```python
from build123d import *

# Parameters (mm, degrees)
ESQUISSE1_W             = 54
ESQUISSE1_H             = 14
ESQUISSE1_W_2           = 50.4
ESQUISSE1_H_2           = 10.4
BOSS_EXTRU_1_DEPTH      = 10
ESQUISSE2_W             = 54
ESQUISSE2_H             = 14
BOSS_EXTRU_2_DEPTH      = 1
ENL_V_MAT_EXTRU_1_DEPTH = 1
ESQUISSE4_W             = 50.4
ESQUISSE4_H             = 10
ENL_V_MAT_EXTRU_2_DEPTH = 1.8


with BuildPart() as part:
    # Esquisse1 → Boss.-Extru.1 (new body)
    with BuildSketch(Plane(origin=(0, 0, 0), x_dir=(1, 0, 0), z_dir=(0, 1, 0))):
        Rectangle(ESQUISSE1_W, ESQUISSE1_H)
        Rectangle(ESQUISSE1_W_2, ESQUISSE1_H_2, mode=Mode.SUBTRACT)
    extrude(amount=BOSS_EXTRU_1_DEPTH)

    # Esquisse2 → Boss.-Extru.2 (add)
    with BuildSketch(Plane(origin=(0, 0, 0), x_dir=(-1, 0, 0), z_dir=(0, -1, 0))):
        Rectangle(ESQUISSE2_W, ESQUISSE2_H)
    extrude(amount=BOSS_EXTRU_2_DEPTH)

    # Esquisse3 → Enlèv. mat.-Extru.1 (cut)
    with BuildSketch(Plane(origin=(0, 0, 0), x_dir=(1, 0, 0), z_dir=(0, 1, 0))):
        with BuildLine():
            Line((-13.3, 0), (-13.3, 7))
            Line((-13.3, 7), (-11.7, 7))
            Line((-11.7, 7), (-11.7, 0))
            ThreePointArc((-11.7, 0), (-12.5, -0.8), (-13.3, 0))
        make_face()
        with BuildLine():
            Line((11.7, 0), (11.7, 7))
            Line((11.7, 7), (13.3, 7))
            Line((13.3, 7), (13.3, 0))
            ThreePointArc((13.3, 0), (12.5, -0.8), (11.7, 0))
        make_face()
    extrude(amount=-ENL_V_MAT_EXTRU_1_DEPTH, mode=Mode.SUBTRACT)

    # Esquisse4 → Enlèv. mat.-Extru.2 (cut)
    with BuildSketch(Plane.XY.offset(-5.2)):
        with Locations((0, 5)):
            Rectangle(ESQUISSE4_W, ESQUISSE4_H)
    extrude(amount=-ENL_V_MAT_EXTRU_2_DEPTH, mode=Mode.SUBTRACT)


solid = part.part
```
Build history of the part. All positions in model axes, mm. A direction names the side the tool comes from. Round coordinates to 2 decimals unless told otherwise and drop trailing zeros. Write each loop counter-clockwise with the first axis right and the second up, starting at its lowest first coordinate (ties: lowest second). Pieces come first, ordered by that corner, then holes. Notation, with made-up numbers: (88, 36.5) - (94, 36.5) arc R20 cw to (94, 55.5) - close; hole circle Ø1 at (27, 57). An arc over 180 degrees is marked (long way). Answer as CSV lines item,"result".
Q1. Pull direction X, two halves, no side cores. Call faces 1 (the flat face through (0, 10, 6)), 2 (the flat face through (27, 5, 0)), 3 (the flat face through (-25.2, 5, -1)), 4 (the flat face through (11.7, -0.5, -3.5)): +X half, -X half, draft (parallel to the pull), parting line (faces both ways), or undercut.
Report:
face 1,"draft"
face 2,"+X half"
face 3,"undercut"
face 4,"undercut"
Q2. Drill centre lines: probe 1 along X at (y, z) = (4.5, 1.5); probe 2 along X at (y, z) = (-0.25, -1.25); probe 3 along Z at (x, y) = (-5.5, 5.25). Where is each one in solid material? Low to high. Write a range as [from, to].
Report:
probe 1,"x = [-27, -25.2], [25.2, 27]"
probe 2,"x = [-27, -13.3], [-11.7, 11.7], [13.3, 27]"
probe 3,"z = [5.2, 7]"
Q3. Cut at C-C (y = 0.75). Write the cut outline in (x, z), and give its area (3 significant figures).
Report:
outline,"(-27, -7) - (-25.2, -7) - (-25.2, 5.2) - (25.2, 5.2) - (25.2, -7) - (27, -7) - (27, 7) - (-27, 7) - close"
area,"141 mm^2"
Q4. Cut at D-D (z = 3.5). Write the cut outline in (x, y).
Report:
outline,"(-27, -1) - (27, -1) - (27, 10) - (25.2, 10) - (25.2, 0) - (-25.2, 0) - (-25.2, 10) - (-27, 10) - close"
Q5. Tool access for faces 5 (the flat face through (-13.3, -0.5, -3.5)), 6 (the flat face through (-26, 2, -7)), 7 (the flat face through (25.2, 5, -1)): list every direction of +Z, -Z, +X, -X, +Y, -Y with a clear straight run to the whole face (end or side of a thin tool).
Report:
face 5,"-Z, +Y, -Y"
face 6,"-Z, +X, -X, +Y, -Y"
face 7,"-Z, +Y"
Q6. Drop flat-ended pins along their axis: pin 1 (3.5 mm diameter, centred on x = 3, z = -1.5, fed in from +Y); pin 2 (3 mm diameter, centred on x = -4.5, y = 7.5, fed in from -Z). Give the stop position or say it passes through.
Report:
pin 1,"stops at y = 0"
pin 2,"stops at z = 5.2"
Q7. Cut at A-A (z = -4.25). Write the cut outline in (x, y).
Report:
outline,"(-27, -1) - (-13.3, -1) - (-13.3, 0) - (-25.2, 0) - (-25.2, 10) - (-27, 10) - close; (-11.7, -1) - (11.7, -1) - (11.7, 0) - (-11.7, 0) - close; (13.3, -1) - (27, -1) - (27, 10) - (25.2, 10) - (25.2, 0) - (13.3, 0) - close"
Q8. Cut at B-B (x = 8.5). Write the cut outline in (y, z).
Report:
outline,"(-1, -7) - (0, -7) - (0, 5.2) - (10, 5.2) - (10, 7) - (-1, 7) - close"
